```python
from build123d import *

# Parameters (mm, degrees)
BOSS_EXTRUDE1_DEPTH = 5.25
BOSS_EXTRUDE2_START = -0.2
BOSS_EXTRUDE2_DEPTH = 1.4
SKETCH2_R           = 1
BOSS_EXTRUDE3_DEPTH = 8.9


with BuildPart() as part:
    # Sketch1 → Boss-Extrude1 (new, symmetric)
    with BuildSketch(Plane(origin=(0, 0, 0), x_dir=(1, 0, 0), z_dir=(0, 1, 0))):
        with BuildLine():
            ThreePointArc((0, -7.735559645), (-0.4049689, -7.287992259), (-0.785238344, -6.8192583))
            ThreePointArc((-0.785238344, -6.8192583), (-7.460228587, -9.979548781), (-14.483869819, -7.69670089))
            Line((-14.483869819, -7.69670089), (-15.25, -8.620304997))
            ThreePointArc((-15.25, -8.620304997), (-7.450762238, -11.181198596), (0, -7.735559645))
        make_face()
        with BuildLine():
            ThreePointArc((14.483869819, -7.69670089), (7.460228587, -9.979548781), (0.785238344, -6.8192583))
            ThreePointArc((0.785238344, -6.8192583), (0.4049689, -7.287992259), (0, -7.735559645))
            ThreePointArc((0, -7.735559645), (7.450762238, -11.181198596), (15.25, -8.620304997))
            Line((15.25, -8.620304997), (14.483869819, -7.69670089))
        make_face()
        with BuildLine():
            Line((0.6, -6.615), (-0.6, -6.615))
            ThreePointArc((-0.6, -6.615), (-0.691915101, -6.71776766), (-0.785238344, -6.8192583))
            ThreePointArc((-0.785238344, -6.8192583), (-0.4049689, -7.287992259), (0, -7.735559645))
            ThreePointArc((0, -7.735559645), (0.4049689, -7.287992259), (0.785238344, -6.8192583))
            ThreePointArc((0.785238344, -6.8192583), (0.691915101, -6.71776766), (0.6, -6.615))
        make_face()
        with BuildLine():
            Line((-0.6, 4.93148467), (-0.6, -4.93148467))
            ThreePointArc((-0.6, -4.93148467), (-0.312960425, -5.406599961), (0, -5.865056097))
            ThreePointArc((0, -5.865056097), (0.312960425, -5.406599961), (0.6, -4.93148467))
            Line((0.6, -4.93148467), (0.6, 4.93148467))
            ThreePointArc((0.6, 4.93148467), (0.312960425, 5.406599961), (0, 5.865056097))
            ThreePointArc((0, 5.865056097), (-0.312960425, 5.406599961), (-0.6, 4.93148467))
        make_face()
        with BuildLine():
            ThreePointArc((0, 7.735559645), (-0.4049689, 7.287992259), (-0.785238344, 6.8192583))
            ThreePointArc((-0.785238344, 6.8192583), (-0.691915101, 6.71776766), (-0.6, 6.615))
            Line((-0.6, 6.615), (0.6, 6.615))
            ThreePointArc((0.6, 6.615), (0.691915101, 6.71776766), (0.785238344, 6.8192583))
            ThreePointArc((0.785238344, 6.8192583), (0.4049689, 7.287992259), (0, 7.735559645))
        make_face()
        with BuildLine():
            ThreePointArc((-14.483869819, 7.69670089), (-7.460228587, 9.979548781), (-0.785238344, 6.8192583))
            ThreePointArc((-0.785238344, 6.8192583), (-0.4049689, 7.287992259), (0, 7.735559645))
            ThreePointArc((0, 7.735559645), (-7.450762238, 11.181198596), (-15.25, 8.620304997))
            Line((-15.25, 8.620304997), (-14.483869819, 7.69670089))
        make_face()
        with BuildLine():
            ThreePointArc((15.25, 8.620304997), (7.450762238, 11.181198596), (0, 7.735559645))
            ThreePointArc((0, 7.735559645), (0.4049689, 7.287992259), (0.785238344, 6.8192583))
            ThreePointArc((0.785238344, 6.8192583), (7.460228587, 9.979548781), (14.483869819, 7.69670089))
            Line((14.483869819, 7.69670089), (15.25, 8.620304997))
        make_face()
        with BuildLine():
            ThreePointArc((0, -5.865056097), (-0.290991494, -6.247235392), (-0.6, -6.615))
            Line((-0.6, -6.615), (0.6, -6.615))
            ThreePointArc((0.6, -6.615), (0.290991494, -6.247235392), (0, -5.865056097))
        make_face()
        with BuildLine():
            ThreePointArc((0, -5.865056097), (0.290991494, -6.247235392), (0.6, -6.615))
            Line((0.6, -6.615), (0.6, -4.93148467))
            ThreePointArc((0.6, -4.93148467), (0.312960425, -5.406599961), (0, -5.865056097))
        make_face()
        with BuildLine():
            ThreePointArc((0, 5.865056097), (0.312960425, 5.406599961), (0.6, 4.93148467))
            Line((0.6, 4.93148467), (0.6, 6.615))
            ThreePointArc((0.6, 6.615), (0.290991494, 6.247235392), (0, 5.865056097))
        make_face()
        with BuildLine():
            Line((-0.6, -4.93148467), (-0.6, -6.615))
            ThreePointArc((-0.6, -6.615), (-0.290991494, -6.247235392), (0, -5.865056097))
            ThreePointArc((0, -5.865056097), (-0.312960425, -5.406599961), (-0.6, -4.93148467))
        make_face()
        with BuildLine():
            Line((-0.6, 6.615), (-0.6, 4.93148467))
            ThreePointArc((-0.6, 4.93148467), (-0.312960425, 5.406599961), (0, 5.865056097))
            ThreePointArc((0, 5.865056097), (-0.290991494, 6.247235392), (-0.6, 6.615))
        make_face()
        with BuildLine():
            Line((0.6, 6.615), (-0.6, 6.615))
            ThreePointArc((-0.6, 6.615), (-0.290991494, 6.247235392), (0, 5.865056097))
            ThreePointArc((0, 5.865056097), (0.290991494, 6.247235392), (0.6, 6.615))
        make_face()
    extrude(amount=BOSS_EXTRUDE1_DEPTH, both=True)

    # Sketch3 → Boss-Extrude2 (add)
    with BuildSketch(Plane.XZ.offset(5.25).offset(BOSS_EXTRUDE2_START)):
        Polygon((0, -7.735559645), (2.39016182, -9.635559645), (-2.39016182, -9.635559645), align=None)
        Polygon((0, 7.735559645), (2.39016182, 9.635559645), (-2.39016182, 9.635559645), align=None)
    extrude(amount=-BOSS_EXTRUDE2_DEPTH)

    # Sketch2 → Boss-Extrude3 (add)
    with BuildSketch(Plane(origin=(0, 5.25, 0), x_dir=(1, 0, 0), z_dir=(0, 1, 0))):
        with Locations((0, 7.443042592)):
            Circle(SKETCH2_R)
        with Locations((0, -7.443042592)):
            Circle(SKETCH2_R)
    extrude(amount=-BOSS_EXTRUDE3_DEPTH)


solid = part.part
```
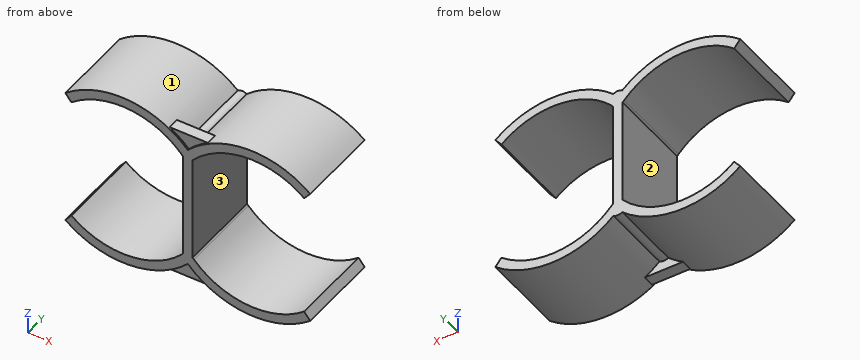
Geometry check sheet. Reference: the model listing, model coordinates, mm. Face numbers are marked on the shaded views. Give positions to 0.01 mm unless a question says otherwise; leave off trailing zeros. Order: outer loops, then holes, each group sorted by start corner. A loop starts at its lowest first (then second) coordinate and runs counter-clockwise, first axis right, second up.
1. Section check A-A, the plane x = -3. Enter the section's corners in (y, z), and give its area (3 significant figures).
2. Section check B-B, the plane y = -4.25. Enter the section's corners in (x, z) (3 decimals).
3. Release check for a two-part mould opening along X. For the marked faces 1, 2 and 3 record: pulls with the +X half, pulls with the -X half, needs draft (parallel to the pull), parting line crosses it, or undercut.
4. Section check D-D, the plane x = 8. Enter the section's corners in (y, z).
5. Section check C-C, the plane z = -6. Enter the section's corners in (x, y).
6. Gauge pin test, flat ends, axial feed: pin 1 Ø1 at (x, z) = (-0.5, 9) entering from -Y; pin 2 Ø0.7 at (x, y) = (-1, -4.5) entering from +Z; pin 3 Ø5 at (y, z) = (-2, 1) entering from -X. Record the tip position at first contact, or that the pin passes through.
7. Thickness scan on L1, parallel to Z at x = -8.5, y = 2; L2, parallel to X at y = -4.5, z = 8.75; L3, parallel to X at y = 4.75, z = -3.5. Record the ranges inside material, lowest first.
Values follow:
1. outline: (-5.25, -9.97) - (5.25, -9.97) - (5.25, -8.6) - (-5.25, -8.6) - close; (-5.25, 8.6) - (5.25, 8.6) - (5.25, 9.97) - (-5.25, 9.97) - close
1. area: 28.8 mm2
2. outline: (-15.25, -8.62) arc R11.2 ccw to (-2.39, -9.636) - (2.39, -9.636) arc R11.2 ccw to (15.25, -8.62) - (14.484, -7.697) arc R10 cw to (0.785, -6.819) arc R10 cw to (0.6, -6.615) - (0.6, 6.615) arc R10 cw to (0.785, 6.819) arc R10 cw to (14.484, 7.697) - (15.25, 8.62) arc R11.2 ccw to (2.39, 9.636) - (-2.39, 9.636) arc R11.2 ccw to (-15.25, 8.62) - (-14.484, 7.697) arc R10 cw to (-0.785, 6.819) arc R10 cw to (-0.6, 6.615) - (-0.6, -6.615) arc R10 cw to (-0.785, -6.819) arc R10 cw to (-14.484, -7.697) - close
3. face 1: undercut
3. face 2: pulls with the -X half
3. face 3: pulls with the +X half
4. outline: (-5.25, -11.2) - (5.25, -11.2) - (5.25, -10) - (-5.25, -10) - close; (-5.25, 10) - (5.25, 10) - (5.25, 11.2) - (-5.25, 11.2) - close
5. outline: (-0.6, -5.25) - (0.6, -5.25) - (0.6, 5.25) - (-0.6, 5.25) - close
6. pin 1: stops at y = -5.05
6. pin 2: stops at z = 9.64
6. pin 3: stops at x = -0.6
7. L1: z = -11.19 to -9.99, 9.99 to 11.19
7. L2: x = -15.09 to -12.94, -3.26 to 3.26, 12.94 to 15.09
7. L3: x = -0.6 to 0.6
